Source: CAD feature listing. Evaluate the final solid. Frame: model axes, mm. A direction names the side the tool comes from. Round coordinates to 2 decimals unless told otherwise and drop trailing zeros. Order: outer loops, then holes, each group sorted by start corner. A loop starts at its lowest first (then second) coordinate and runs counter-clockwise, first axis right, second up. Notation, with made-up numbers: M -5,-18 L 26,-18 A20 cw 26,9 Z; hole C 22,59.25 d10. An arc over 180 degrees is marked long. Answer in a Markdown table with one row per item. Add a question column.
```python
from build123d import *

# Parameters (mm, degrees)
F1_DEPTH = 15


with BuildPart() as f1:
    # F0 (on Top) → F1 (new body)
    with BuildSketch(Plane.XY):
        with BuildLine():
            ThreePointArc((-5, -42), (-4.12132, -44.12132), (-2, -45))
            Line((-2, -45), (0, -45))
            Line((0, -45), (0, 0))
            Line((0, 0), (5, 0))
            Line((5, 0), (5, 25))
            Line((5, 25), (11, 25))
            Line((11, 25), (11, 22))
            Line((11, 22), (16, 22))
            Line((16, 22), (16, 27))
            ThreePointArc((16, 27), (15.12132, 29.12132), (13, 30))
            Line((13, 30), (3.459412, 30))
            ThreePointArc((3.459412, 30), (1.557445, 29.320026), (0.51767, 27.588348))
            Line((0.51767, 27.588348), (-4.941742, 0.29129))
            ThreePointArc((-4.941742, 0.29129), (-4.9854, -0.001446), (-5, -0.297059))
            Line((-5, -0.297059), (-5, -42))
        make_face()
    extrude(amount=F1_DEPTH)


solid = f1.part
```
(1) Pin query (flat end, axial travel): pin 1 (5 mm diameter, centred on x = -1, z = 8.5, fed in from +Y); pin 2 (2.5 mm diameter, centred on y = 24, z = 4.5, fed in from -X); pin 3 (2.5 mm diameter, centred on x = 3.5, z = 5.5, fed in from -Y). Return the tip coordinate at first contact, or that it passes through.
(2) Line query: line 1 (X direction, y = 23.5, z = 1.75); line 2 (X direction, y = -12, z = 7.5); line 3 (Y direction, x = 3.25, z = 7). Output: solid intervals per line, ascending. Write a range as from..to.
(3) Cut plane C-C (x = 7.75). Return loops of the section in (y, z).
(4) Cut plane A-A (z = 8.25). Return loops of the section in (x, y), and give its area (3 significant figures).
(5) Access query for faces 1 (the face through (16, 24, 7)), 2 (the face through (2, 0, 7)), 3 (the face through (8, 25, 7)). Directions: +Z, -Z, +X, -X, +Y, -Y. A direction counts if a zero-diameter tool reaches every point of the face in a straight line with its end or side. Return the directions, or none.
(6) Cut plane B-B (y = 21). Return loops of the section in (x, z).
(7) Draft query along X for faces 4 (the face through (-2.174, 14.131, 7.395)), 5 (the face through (0, -23, 7)), 6 (the face through (11, 24, 7)), 7 (the face through (8, 30, 7)). Return one class per face: +X half, -X half, draft (parallel to the pull), parting line (faces both ways), or undercut.
Answer list:
| question | item | result |
|---|---|---|
| 1 | pin 1 | y = 29.27 |
| 1 | pin 2 | x = -0.45 |
| 1 | pin 3 | y = 0 |
| 2 | line 1 | -0.3..5, 11..16 |
| 2 | line 2 | -5..0 |
| 2 | line 3 | 0..29.99 |
| 3 | outline | M 25,0 L 30,0 L 30,15 L 25,15 Z |
| 4 | outline | M -5,-42 A3 ccw -2,-45 L 0,-45 L 0,0 L 5,0 L 5,25 L 11,25 L 11,22 L 16,22 L 16,27 A3 ccw 13,30 L 3.46,30 A3 ccw 0.52,27.59 L -4.94,0.29 A3 ccw -5,-0.3 Z |
| 4 | area | 500 mm² |
| 5 | face 1 | +Z, -Z, +X, +Y, -Y |
| 5 | face 2 | +Z, -Z, +X, -Y |
| 5 | face 3 | +Z, -Z, -Y |
| 6 | outline | M -0.8,0 L 5,0 L 5,15 L -0.8,15 Z |
| 7 | face 4 | -X half |
| 7 | face 5 | +X half |
| 7 | face 6 | undercut |
| 7 | face 7 | draft |
